```python
from build123d import *

# Parameters (mm, degrees)
SKETCH1_R           = 203.2
BOSS_EXTRUDE1_DEPTH = 12.7
BOSS_EXTRUDE1_DRAFT = -63.999999999
SKETCH2_R           = 183.871225213
CUT_EXTRUDE1_DEPTH  = 5.08
CUT_EXTRUDE1_DRAFT  = -83.999999999
FILLET1_R           = 2.54
SCALE1_SCALE        = 0.582


with BuildPart() as part:
    # Sketch1 → Boss-Extrude1 (with draft: the straight prism first)
    with BuildSketch(Plane(origin=(0, 0, 0), x_dir=(1, 0, 0), z_dir=(0, 1, 0))):
        Circle(SKETCH1_R)
    extrude(amount=BOSS_EXTRUDE1_DEPTH)
    # Boss-Extrude1: the draft: its side faces are tilted about the plane it starts from
    boss_extrude1_sides = [part.faces().sort_by_distance(p)[0] for p in [
        (-203.2, 6.35, 0),
    ]]
    draft(boss_extrude1_sides, Plane(origin=(0, 0, 0), x_dir=(1, 0, 0), z_dir=(0, 1, 0)), BOSS_EXTRUDE1_DRAFT)


with BuildPart() as cut_extrude1_tool:
    # Sketch2 → Cut-Extrude1 (with draft: the straight prism first)
    with BuildSketch(Plane(origin=(0, 12.7, 0), x_dir=(1, 0, 0), z_dir=(0, 1, 0))):
        Circle(SKETCH2_R)
    extrude(amount=-CUT_EXTRUDE1_DEPTH)
    # Cut-Extrude1: the draft: its side faces are tilted about the plane it starts from
    cut_extrude1_sides = [cut_extrude1_tool.faces().sort_by_distance(p)[0] for p in [
        (-183.871225213, 10.16, 0),
    ]]
    draft(cut_extrude1_sides, Plane(origin=(0, 12.7, 0), x_dir=(1, 0, 0), z_dir=(0, 1, 0)), CUT_EXTRUDE1_DRAFT)


with BuildPart() as part_1:
    add(part.part)

    # Cut-Extrude1: cut by cut_extrude1_tool
    add(cut_extrude1_tool.part, mode=Mode.SUBTRACT)

    # Fillet1
    fillet1_edges = [part_1.edges().sort_by_distance(p)[0] for p in [
        (-229.238858787, 12.7, 0),
        (-135.53825379, 7.62, 0),
        (-183.871225213, 12.7, 0),
    ]]
    fillet(fillet1_edges, radius=FILLET1_R)


with BuildPart() as part_2:
    # Scale1: scaled about (0, 5.422815949, 0)
    add(part_1.part.scale(SCALE1_SCALE).moved(Location((0, 2.266737067, 0))))


solid = part_2.part
```
The model under review builds one solid part; all positions refer to its coordinate system, in mm. Coordinates: 2 decimals unless noted, no trailing zeros. Write each loop counter-clockwise with the first axis right and the second up, starting at its lowest first coordinate (ties: lowest second). Pieces come first, ordered by that corner, then holes. Notation, with made-up numbers: (35, 73.5) - (75, 73.5) arc R24 cw to (75, 88.5) - close; hole circle Ø4 at (9, 42). An arc over 180 degrees is marked (long way). Answer in a Markdown table with one row per item. Add a question column.
Q1. To check wall thickness, follow line 1 along Y through (x, z) = (-12, 15); line 2 along Y through (x, z) = (-63, 86); line 3 along X through (y, z) = (3, 9.5). State the ranges of each line that lie inside material, in increasing order. Write a range as from..to.
Q2. Consider section B-B on z = 0. Give the boundary of the cut face in (x, y), then the cut area to 3 significant figures.
Q3. Draft analysis for pull direction Z (two halves, no side actions). For faces 1 (the face through (-1, 6.702, -1)), 2 (the face through (-2, 2.267, -2)), 3 (the face through (-15.45, 2.49, -117.71)), state which applies: +Z half, -Z half, draft (parallel to the pull), parting line (faces both ways), or undercut.
Q4. Consider section A-A on x = 0. Give the boundary of the cut face in (y, z), then the cut area to 3 significant figures.
Q5. Consider section C-C on y = 5.5. Give the boundary of the cut face in (x, z).
Q6. Clearance check with flat-ended pins moving along their axes: pin 1 (1 mm diameter, centred on x = -29, y = 7, fed in from +Z); pin 2 (1.5 mm diameter, centred on x = -2, z = -31.5, fed in from +Y); pin 3 (1 mm diameter, centred on x = -60.5, y = 3.5, fed in from +Z). State where each tip first meets the part, or that it passes through.
Answers below:
| question | item | result |
|---|---|---|
| 1 | line 1 | 2.27..6.7 |
| 1 | line 2 | 2.27..9.62 |
| 1 | line 3 | -119.39..119.39 |
| 2 | outline | (-127.66, 6.85) - (-118.26, 2.27) - (118.26, 2.27) - (127.66, 6.85) arc R1.48 ccw to (127.01, 9.66) - (107.09, 9.66) arc R1.48 ccw to (106.94, 9.65) - (78.96, 6.71) arc R1.48 cw to (78.81, 6.7) - (-78.81, 6.7) arc R1.48 cw to (-78.96, 6.71) - (-106.94, 9.65) arc R1.48 ccw to (-107.09, 9.66) - (-127.01, 9.66) arc R1.48 ccw to start |
| 2 | area | 1,300 mm² |
| 3 | face 1 | undercut |
| 3 | face 2 | draft |
| 3 | face 3 | parting line |
| 4 | outline | (2.27, -118.26) - (6.85, -127.66) arc R1.48 ccw to (9.66, -127.01) - (9.66, -107.09) arc R1.48 ccw to (9.65, -106.94) - (6.71, -78.96) arc R1.48 cw to (6.7, -78.81) - (6.7, 78.81) arc R1.48 cw to (6.71, 78.96) - (9.65, 106.94) arc R1.48 ccw to (9.66, 107.09) - (9.66, 127.01) arc R1.48 ccw to (6.85, 127.66) - (2.27, 118.26) - close |
| 4 | area | 1,300 mm² |
| 5 | outline | circle Ø249.78 at (0, 0) |
| 6 | pin 1 | z = 125.03 |
| 6 | pin 2 | y = 6.7 |
| 6 | pin 3 | z = 105.76 |
